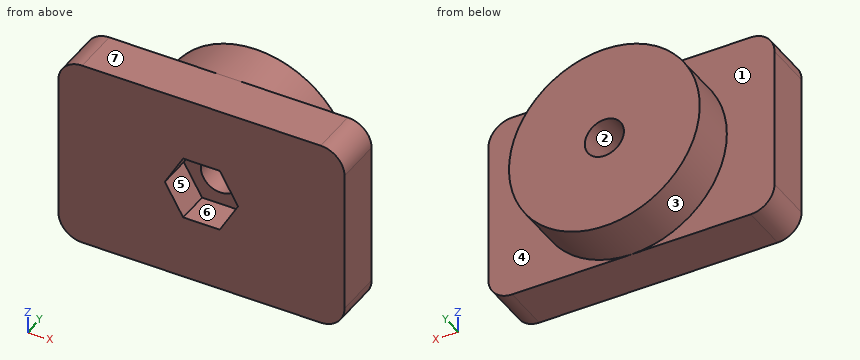
```python
from build123d import *

# Parameters (mm, degrees)
SKETCH1_W           = 60
SKETCH1_H           = 40
BOSS_EXTRUDE1_DEPTH = 10
SKETCH2_R           = 20
BOSS_EXTRUDE2_DEPTH = 10
SKETCH4_R           = 4.1
CUT_EXTRUDE1_DEPTH  = 42.231056256
FILLET1_R           = 5
CUT_EXTRUDE2_DEPTH  = 7


with BuildPart() as part:
    # Sketch1 → Boss-Extrude1 (new body)
    with BuildSketch(Plane(origin=(0, 0, 0), x_dir=(1, 0, 0), z_dir=(0, 1, 0))):
        Rectangle(SKETCH1_W, SKETCH1_H)
    extrude(amount=BOSS_EXTRUDE1_DEPTH)

    # Sketch2 → Boss-Extrude2 (add)
    with BuildSketch(Plane(origin=(0, 10, 0), x_dir=(1, 0, 0), z_dir=(0, 1, 0))):
        with Locations(Location((0, 0, 0), (0, 0, 270))):
            Circle(SKETCH2_R)
    extrude(amount=BOSS_EXTRUDE2_DEPTH)

    # Sketch4 → Cut-Extrude1 (cut, through all)
    with BuildSketch(Plane(origin=(0, 20, 0), x_dir=(1, 0, 0), z_dir=(0, 1, 0))):
        with Locations(Location((0, 0, 0), (0, 0, 270))):
            Circle(SKETCH4_R)
    extrude(amount=-CUT_EXTRUDE1_DEPTH, mode=Mode.SUBTRACT)

    # Fillet1
    fillet1_edges = [part.edges().sort_by_distance(p)[0] for p in [
        (-30, 5, -20),
        (30, 5, -20),
        (30, 5, 20),
        (-30, 5, 20),
    ]]
    fillet(fillet1_edges, radius=FILLET1_R)

    # Sketch5 → Cut-Extrude2 (cut)
    with BuildSketch(Plane.XZ):
        Polygon((-7.67875858, 0), (-3.83937929, -6.65), (3.83937929, -6.65), (7.67875858, 0), (3.83937929, 6.65), (-3.83937929, 6.65), align=None)
    extrude(amount=-CUT_EXTRUDE2_DEPTH, mode=Mode.SUBTRACT)


solid = part.part
```
Verification items for the finished model (mm, model axes). Face numbers are marked on the shaded views. A direction names the side the tool comes from. Coordinates: 2 decimals unless noted, no trailing zeros. Write each loop counter-clockwise with the first axis right and the second up, starting at its lowest first coordinate (ties: lowest second). Pieces come first, ordered by that corner, then holes. Notation, with made-up numbers: (11.25, -9.5) - (57.25, -9.5) arc R8 ccw to (57.25, -1.5) - close; hole circle Ø11 at (85, 30.5). An arc over 180 degrees is marked (long way). Write item = value, one per line.
Q1. Cross-section at D-D (x = 12). Enter the section's corners in (y, z), plus the area to 3 significant figures.
Answer:
outline = (0, -20) - (10, -20) - (10, -16) - (20, -16) - (20, 16) - (10, 16) - (10, 20) - (0, 20) - close
area = 720 mm²
Q2. Cross-section at C-C (z = 12). Enter the section's corners in (x, y).
Answer:
outline = (-30, 0) - (30, 0) - (30, 10) - (16, 10) - (16, 20) - (-16, 20) - (-16, 10) - (-30, 10) - close
Q3. Mould release check, pull along Z, two halves, no side actions. Record for the marked faces 4, 5, 6 and 7: released by +Z, released by -Z, zero draft, split by the parting line, or undercut.
Answer:
face_4 = zero draft
face_5 = undercut
face_6 = undercut
face_7 = released by +Z
Q4. Cross-section at A-A (x = 2.5). Enter the section's corners in (y, z), plus the area to 3 significant figures.
Answer:
outline = (0, -20) - (10, -20) - (10, -19.84) - (20, -19.84) - (20, -3.25) - (7, -3.25) - (7, -6.65) - (0, -6.65) - close; (0, 6.65) - (7, 6.65) - (7, 3.25) - (20, 3.25) - (20, 19.84) - (10, 19.84) - (10, 20) - (0, 20) - close
area = 619 mm²
Q5. Material ranges on L1, parallel to X at y = 11.5, z = 0; L2, parallel to Z at x = 2, y = 6.75; L3, parallel to Y at x = 22.5, z = -4.5, recorded low to high. Write a range as from..to.
Answer:
L1 = -20..-4.1, 4.1..20
L2 = -20..-6.65, 6.65..20
L3 = 0..10
Q6. Access from +Z, -Z, +X, -X, +Y, -Y to the whole of each face (thin tool, end or side, straight path). Record for the marked faces 1, 2 and 3.
Answer:
face_1 = -X, +Y
face_2 = +Y, -Y
face_3 = +Y
Q7. Cross-section at B-B (y = 5.25). Enter the section's corners in (x, z), plus the area to 3 significant figures.
Answer:
outline = (-30, -15) arc R5 ccw to (-25, -20) - (25, -20) arc R5 ccw to (30, -15) - (30, 15) arc R5 ccw to (25, 20) - (-25, 20) arc R5 ccw to (-30, 15) - close; hole (-7.68, 0) - (-3.84, -6.65) - (3.84, -6.65) - (7.68, 0) - (3.84, 6.65) - (-3.84, 6.65) - close
area = 2,230 mm²
Q8. Go/stop test with flat-tipped pins: pin 1 Ø8 at (x, y) = (-16, 16.5) entering from +Z; pin 2 Ø4 at (x, z) = (1.5, -3) entering from -Y; pin 3 Ø3 at (x, y) = (14, 18) entering from +Z. Record where each tip stops, or that it passes through.
Answer:
pin_1 = 16
pin_2 = 7
pin_3 = 15.61
